```python
from build123d import *

# Parameters (mm, degrees)
F0_W          = 127
F0_H          = 2100
F1_DEPTH      = 127
F2_DEPTH      = 127
F2_DEPTH_BACK = 1000
F0_W_2        = 10.0161342862
F0_H_2        = 803.2517696619
F3_DEPTH      = 586


with BuildPart() as f1:
    # F0 (on Front) → F1 (new body)
    with BuildSketch(Plane.XZ):
        Rectangle(F0_W, F0_H)
        Polygon((-10.3423068728, -835), (0.7857291494, -835), (11.9137651715, -835), (11.9137651715, -810), (21.7857291494, -810), (21.7857291494, -850), (25, -850), (25, -1000), (-25, -1000), (-25, -850), (-20.2142708506, -850), (-20.2142708506, -810), (-10.3423068728, -810), align=None, mode=Mode.SUBTRACT)
        Polygon((-10.0161342919, 895.125884831), (-2.774e-07, 895.125884831), (10.0161340088, 895.125884831), (10.0161340088, 91.874115169), (-5.7e-09, 91.874115169), (-10.0161342919, 91.874115169), align=None, mode=Mode.SUBTRACT)
        Polygon((-11.5747122988, 90), (-5.1e-09, 90), (10.6813597456, 90), (10.6813597456, 115), (20.5533237234, 115), (20.5533237234, 75), (25.5, 75), (25.5, -13), (21.3999971747, -13), (21.3999971747, -53), (11.5280331969, -53), (11.5280331969, -28), (0.7857291494, -28), (-10.7280388474, -28), (-10.7280388474, -53), (-20.6000028253, -53), (-20.6000028253, -13), (-25.5, -13), (-25.5, 75), (-21.4466762766, 75), (-21.4466762766, 115), (-11.5747122988, 115), align=None, mode=Mode.SUBTRACT)
        Polygon((25.5, 1000), (25.5, 912), (20.9999997169, 912), (20.9999997169, 872), (11.1280357391, 872), (11.1280357391, 897), (-2.78e-07, 897), (-11.1280363053, 897), (-11.1280363053, 872), (-21.0000002831, 872), (-21.0000002831, 912), (-25.5, 912), (-25.5, 1000), align=None, mode=Mode.SUBTRACT)
        Polygon((20.9999997169, 872), (20.9999997169, 912), (-2.831e-07, 912), (-2.78e-07, 897), (11.1280357391, 897), (11.1280357391, 872), align=None)
        Polygon((-2.78e-07, 897), (-2.831e-07, 912), (-21.0000002831, 912), (-21.0000002831, 872), (-11.1280363053, 872), (-11.1280363053, 897), align=None)
        Polygon((21.3999971747, -53), (21.3999971747, -13), (0.7857291494, -13), (0.7857291494, -28), (11.5280331969, -28), (11.5280331969, -53), align=None)
        Polygon((0.7857291494, -13), (-20.6000028253, -13), (-20.6000028253, -53), (-10.7280388474, -53), (-10.7280388474, -28), (0.7857291494, -28), align=None)
    extrude(amount=F1_DEPTH)

    # F0 (on Front) → F2 (join, two sides)
    with BuildSketch(Plane.XZ) as f2_sk:
        Polygon((11.9137651715, -835), (0.7857291494, -835), (0.7857291494, -850), (21.7857291494, -850), (21.7857291494, -810), (11.9137651715, -810), align=None)
        Polygon((0.7857291494, -850), (0.7857291494, -835), (-10.3423068728, -835), (-10.3423068728, -810), (-20.2142708506, -810), (-20.2142708506, -850), align=None)
        Polygon((10.6813597456, 90), (-5.1e-09, 90), (0, 75), (20.5533237234, 75), (20.5533237234, 115), (10.6813597456, 115), align=None)
        Polygon((0, 75), (-5.1e-09, 90), (-11.5747122988, 90), (-11.5747122988, 115), (-21.4466762766, 115), (-21.4466762766, 75), align=None)
        Polygon((20.9999997169, 912), (25.5, 912), (25.5, 1000), (-25.5, 1000), (-25.5, 912), (-21.0000002831, 912), (-2.831e-07, 912), align=None)
        Polygon((20.9999997169, 872), (20.9999997169, 912), (-2.831e-07, 912), (-2.78e-07, 897), (11.1280357391, 897), (11.1280357391, 872), align=None)
        Polygon((-2.78e-07, 897), (-2.831e-07, 912), (-21.0000002831, 912), (-21.0000002831, 872), (-11.1280363053, 872), (-11.1280363053, 897), align=None)
        Polygon((20.5533237234, 75), (0, 75), (-21.4466762766, 75), (-25.5, 75), (-25.5, -13), (-20.6000028253, -13), (0.7857291494, -13), (21.3999971747, -13), (25.5, -13), (25.5, 75), align=None)
        Polygon((21.3999971747, -53), (21.3999971747, -13), (0.7857291494, -13), (0.7857291494, -28), (11.5280331969, -28), (11.5280331969, -53), align=None)
        Polygon((0.7857291494, -13), (-20.6000028253, -13), (-20.6000028253, -53), (-10.7280388474, -53), (-10.7280388474, -28), (0.7857291494, -28), align=None)
        Polygon((21.7857291494, -850), (0.7857291494, -850), (-20.2142708506, -850), (-25, -850), (-25, -1000), (25, -1000), (25, -850), align=None)
    extrude(amount=-F2_DEPTH)
    extrude(f2_sk.sketch, amount=F2_DEPTH_BACK)

    # F0 (on Front) → F3 (join)
    with BuildSketch(Plane.XZ):
        with Locations((5.0080668657, 493.5)):
            Rectangle(F0_W_2, F0_H_2)
        with Locations((-5.0080671488, 493.5)):
            Rectangle(F0_W_2, F0_H_2)
    extrude(amount=F3_DEPTH)


solid = f1.part
```
Geometry: final body of the model. Coordinates: model frame, mm. A direction names the side the tool comes from. Give positions to 0.01 mm unless a question says otherwise; leave off trailing zeros. Loops run counter-clockwise (first coordinate to the right, second up) from the corner with the lowest first, then second, coordinate; pieces in that order, holes last. Notation, with made-up numbers: (79.5, 24) - (100.5, 24) arc R20 ccw to (100.5, 59) - close; hole circle Ø1 at (58.25, 0.25). An arc over 180 degrees is marked (long way). Answer as CSV lines item,"result". Start each with the question number.
(1) Ray query, line 1 along Z through (x, y) = (-2.5, -910.5); line 2 along Z through (x, y) = (-9, -217); line 3 along Z through (x, y) = (-18, -145.5). Return the intervals inside material, ascending. Write a range as [from, to].
(2) Pin query (flat end, axial travel): P1, Ø12.5, axis at y = 55.5, z = 101.5, coming from the +X side; P2, Ø11, axis at x = -17.5, y = 63.5, coming from the +Z side; P3, Ø5, axis at x = -48, z = 237, coming from the -Y side. Return the tip coordinate at first contact, or that it passes through.
(3) Section query C-C (z = 654). Output: boundary loops of the cut face in (x, y), and give its area (3 significant figures).
(4) Mould query, pull axis Z, two halves, no side actions, for faces 1 (the face through (-10.016, -353, 488)), 2 (the face through (27, -127, 15)), 3 (the face through (-25, 63, -924)), 4 (the face through (-1, -63, 1050)). Classes: +Z half, -Z half, draft (parallel to the pull), parting line (faces both ways), or undercut.
(5) Reachability of faces 5 (the face through (0, -557, 1000)), 6 (the face through (-21.447, 63, 95)), 7 (the face through (-25.5, 63, 957)), 8 (the face through (21.786, -557, -830)) from +Z, -Z, +X, -X, +Y, -Y: full face, straight path, thin tool, end or side. Return the list, or none.
(6) Section query B-B (y = -907.5). Give the number of separate pieces and of enclosed holes in the cut face, and give its area (3 significant figures).
(7) Section query A-A (z = -873). Output: boundary loops of the cut face in (x, y).
Worked answers:
1,line 1,"z = [-1000, -835], [-28, 90], [897, 1000]"
1,line 2,"z = [-1000, -835], [-28, 90], [91.87, 895.13], [897, 1000]"
1,line 3,"z = [-1000, -810], [-53, 115], [872, 1000]"
2,P1,"stops at x = 20.55"
2,P2,"stops at z = 1000"
2,P3,"stops at y = -127"
3,outline,"(-63.5, -127) - (-10.02, -127) - (-10.02, -586) - (10.02, -586) - (10.02, -127) - (63.5, -127) - (63.5, 0) - (-63.5, 0) - close"
3,area,"25,300 mm^2"
4,face 1,"undercut"
4,face 2,"undercut"
4,face 3,"draft"
4,face 4,"+Z half"
5,face 5,"+Z, +X, -X, -Y"
5,face 6,"-X, +Y"
5,face 7,"+Z, -Z, -X, +Y"
5,face 8,"+X, -Y"
6,separate pieces,"3"
6,enclosed holes,"0"
6,area,"21,000 mm^2"
7,outline,"(-63.5, -127) - (-25, -127) - (-25, -1000) - (25, -1000) - (25, -127) - (63.5, -127) - (63.5, 0) - (25, 0) - (25, 127) - (-25, 127) - (-25, 0) - (-63.5, 0) - close"
